```python
from build123d import *

# Parameters (mm, degrees)
SKETCH_W     = 28
SKETCH_H     = 28
PAD_DEPTH    = 1
PAD001_DEPTH = 4.2
SKETCH002_W  = 8
SKETCH002_H  = 4
PAD002_DEPTH = 3
SKETCH003_W  = 25
SKETCH003_H  = 18
PAD003_DEPTH = 2
SKETCH004_R  = 2.236068
PAD004_DEPTH = 1.5
SKETCH005_R  = 0.5
POCKET_DEPTH = 5.201


with BuildPart() as part:
    # Sketch → Pad (new body)
    with BuildSketch(Plane.XY):
        Rectangle(SKETCH_W, SKETCH_H)
    extrude(amount=PAD_DEPTH)

    # Sketch001 (on Face6 of Pad) → Pad001 (join)
    with BuildSketch(Plane.XY.offset(1)):
        with BuildLine():
            Line((-11, 12.5), (11, 12.5))
            ThreePointArc((12.5, 11), (12.06066, 12.06066), (11, 12.5))
            Line((12.5, 11), (12.5, -11))
            ThreePointArc((11, -12.5), (12.06066, -12.06066), (12.5, -11))
            Line((11, -12.5), (-11, -12.5))
            ThreePointArc((-12.5, -11), (-12.06066, -12.06066), (-11, -12.5))
            Line((-12.5, -11), (-12.5, 11))
            ThreePointArc((-11, 12.5), (-12.06066, 12.06066), (-12.5, 11))
        make_face()
    extrude(amount=PAD001_DEPTH)

    # Sketch002 (on Face4 of Pad001) → Pad002 (join)
    with BuildSketch(Plane(origin=(0, 0, 0), x_dir=(1, 0, 0), z_dir=(0, 0, -1))):
        with Locations((0, -9)):
            Rectangle(SKETCH002_W, SKETCH002_H)
    extrude(amount=PAD002_DEPTH)

    # Sketch003 (on Face4 of Pad002) → Pad003 (join)
    with BuildSketch(Plane(origin=(0, 0, 0), x_dir=(1, 0, 0), z_dir=(0, 0, -1))):
        with Locations((0, 3.5)):
            Rectangle(SKETCH003_W, SKETCH003_H)
    extrude(amount=PAD003_DEPTH)

    # Sketch004 (on Face4 of Pad003) → Pad004 (join)
    with BuildSketch(Plane(origin=(0, 0, 0), x_dir=(1, 0, 0), z_dir=(0, 0, -1))):
        with Locations((9, -10)):
            Circle(SKETCH004_R)
    extrude(amount=PAD004_DEPTH)

    # Sketch005 (on Face4 of Pad004) → Pocket (cut, through all)
    with BuildSketch(Plane(origin=(0, 0, 0), x_dir=(1, 0, 0), z_dir=(0, 0, -1))):
        with Locations((-5, -13.37)):
            Circle(SKETCH005_R)
        with Locations((-3, -13.37)):
            Circle(SKETCH005_R)
        with Locations((-1, -13.37)):
            Circle(SKETCH005_R)
        with Locations((1, -13.37)):
            Circle(SKETCH005_R)
        with Locations((3, -13.37)):
            Circle(SKETCH005_R)
        with Locations((5, -13.37)):
            Circle(SKETCH005_R)
    extrude(amount=-POCKET_DEPTH, mode=Mode.SUBTRACT)


solid = part.part
```
Can you work these out from the model? Positions are in its coordinate system, mm. A direction names the side the tool comes from. Coordinates: 2 decimals unless noted, no trailing zeros. Order: outer loops, then holes, each group sorted by start corner. A loop starts at its lowest first (then second) coordinate and runs counter-clockwise, first axis right, second up.
1. I need wall thicknesses on line 1 (X direction, y = -7.25, z = 4); line 2 (Z direction, x = -5.5, y = 3.25); line 3 (Z direction, x = 4.5, y = 8). Which ranges of each line are inside material? Lowest first, please.
2. I'm going to push flat-ended pins straight in: pin 1 (3 mm diameter, centred on y = 10, z = 3.5, fed in from -X); pin 2 (4.5 mm diameter, centred on y = 3, z = 3.5, fed in from +X); pin 3 (3.5 mm diameter, centred on x = -3, z = 4, fed in from -Y); pin 4 (2 mm diameter, centred on y = -1.5, z = -0.5, fed in from +X). Where does each tip first touch, or does it pass through?
3. Thinking about a two-plate mould opening in X: for faces 6 (the face through (5.231, 13.814, 0.493)), 7 (the face through (-2.769, 13.814, 0.493)), 8 (the face through (9, 10, -1.5)), 9 (the face through (-12.07, -12.05, 3.07)), which applies, +X half, -X half, draft (parallel to the pull), parting line (faces both ways), or undercut?
4. If we section it at C-C (z = 3): Please give me the cut outline in (x, y).
5. If we section it at A-A (y = 13.37): Please give me the cut outline in (x, z), then the cut area to 3 significant figures.
6. If we section it at B-B (x = 1): Please give me the cut outline in (y, z).
7. For faces 1 (the face through (0, -12.5, 3)), 2 (the face through (0, 7, -1)), 3 (the face through (-4, 9, -1)), 4 (the face through (12.05, -12.07, 3.07)), 5 (the face through (0, -12.5, -1)), which set-ups out of +Z, -Z, +X, -X, +Y, -Y let a thin tool reach every point of the face, with its end or its side?
8. If we section it at D-D (z = -0.75): Please give me the cut outline in (x, y), then the cut area to 3 significant figures.
Entries:
1. line 1: x = -12.5 to 12.5
1. line 2: z = -2 to 5.2
1. line 3: z = 0 to 5.2
2. pin 1: stops at x = -12.5
2. pin 2: stops at x = 12.5
2. pin 3: stops at y = -12.5
2. pin 4: stops at x = 14
3. face 6: undercut
3. face 7: undercut
3. face 8: draft
3. face 9: -X half
4. outline: (-12.5, -11) arc R1.5 ccw to (-11, -12.5) - (11, -12.5) arc R1.5 ccw to (12.5, -11) - (12.5, 11) arc R1.5 ccw to (11, 12.5) - (-11, 12.5) arc R1.5 ccw to (-12.5, 11) - close
5. outline: (-14, 0) - (-5.5, 0) - (-5.5, 1) - (-14, 1) - close; (-4.5, 0) - (-3.5, 0) - (-3.5, 1) - (-4.5, 1) - close; (-2.5, 0) - (-1.5, 0) - (-1.5, 1) - (-2.5, 1) - close; (-0.5, 0) - (0.5, 0) - (0.5, 1) - (-0.5, 1) - close; (1.5, 0) - (2.5, 0) - (2.5, 1) - (1.5, 1) - close; (3.5, 0) - (4.5, 0) - (4.5, 1) - (3.5, 1) - close; (5.5, 0) - (14, 0) - (14, 1) - (5.5, 1) - close
5. area: 22.0 mm2
6. outline: (-14, 0) - (-12.5, 0) - (-12.5, -2) - (5.5, -2) - (5.5, 0) - (7, 0) - (7, -3) - (11, -3) - (11, 0) - (12.87, 0) - (12.87, 1) - (12.5, 1) - (12.5, 5.2) - (-12.5, 5.2) - (-12.5, 1) - (-14, 1) - close; (13.87, 0) - (14, 0) - (14, 1) - (13.87, 1) - close
7. face 1: +Z, +X, -X, -Y
7. face 2: -Z, +X, -X
7. face 3: -Z, -X, +Y
7. face 4: +Z, +X, -Y
7. face 5: -Z, +X, -X, -Y
8. outline: (-12.5, -12.5) - (12.5, -12.5) - (12.5, 5.5) - (-12.5, 5.5) - close; (-4, 7) - (4, 7) - (4, 11) - (-4, 11) - close; circle Ø4.47 at (9, 10)
8. area: 498 mm2
